```python
from build123d import *

# Parameters (mm, degrees)
SKETCH2_W           = 226.3
SKETCH2_H           = 100
BOSS_EXTRUDE1_DEPTH = 183
SKETCH4_OUTSIDE_W   = 316.656
SKETCH4_OUTSIDE_H   = 190.356
SKETCH4_OUTSIDE_W_2 = 8.5
SKETCH4_OUTSIDE_H_2 = 8.5
CUT_EXTRUDE1_DEPTH  = 6
SKETCH5_W           = 209.3
SKETCH5_H           = 114
CUT_EXTRUDE2_DEPTH  = 238.259188442
SKETCH6_W           = 83
SKETCH6_H           = 114
CUT_EXTRUDE3_DEPTH  = 296.29762952
EXTRUDE_THIN1_START = -2.5
EXTRUDE_THIN1_DEPTH = 3.5
EXTRUDE_THIN2_START = -2.5
EXTRUDE_THIN2_DEPTH = 3.5
CIRPATTERN1_COUNT   = 2


with BuildPart() as part:
    # Sketch2 → Boss-Extrude1 (new, symmetric)
    with BuildSketch(Plane(origin=(0, 0, 0), x_dir=(1, 0, 0), z_dir=(0, 1, 0))):
        Rectangle(SKETCH2_W, SKETCH2_H)
    extrude(amount=BOSS_EXTRUDE1_DEPTH, both=True)

    # Sketch4 outside → Cut-Extrude1 (cut)
    with BuildSketch(Plane.XZ.offset(183)):
        Rectangle(SKETCH4_OUTSIDE_W, SKETCH4_OUTSIDE_H)
        with Locations((-108.9, 45.75)):
            Rectangle(SKETCH4_OUTSIDE_W_2, SKETCH4_OUTSIDE_H_2, mode=Mode.SUBTRACT)
        with Locations((-108.9, -45.75)):
            Rectangle(SKETCH4_OUTSIDE_W_2, SKETCH4_OUTSIDE_H_2, mode=Mode.SUBTRACT)
        with Locations((108.9, -45.75)):
            Rectangle(SKETCH4_OUTSIDE_W_2, SKETCH4_OUTSIDE_H_2, mode=Mode.SUBTRACT)
        with Locations((108.9, 45.75)):
            Rectangle(SKETCH4_OUTSIDE_W_2, SKETCH4_OUTSIDE_H_2, mode=Mode.SUBTRACT)
    cut_extrude1 = extrude(amount=-CUT_EXTRUDE1_DEPTH, mode=Mode.SUBTRACT)

    # Mirror1: Cut-Extrude1 across plane
    add(cut_extrude1.mirror(Plane.ZX), mode=Mode.SUBTRACT)

    # Sketch5 → Cut-Extrude2 (cut, through all)
    with BuildSketch(Plane.XY.offset(50)):
        with Locations((0, 117)):
            Rectangle(SKETCH5_W, SKETCH5_H)
        with Locations((0, -117)):
            Rectangle(SKETCH5_W, SKETCH5_H)
        Rectangle(SKETCH5_W, SKETCH5_H)
    extrude(amount=-CUT_EXTRUDE2_DEPTH, mode=Mode.SUBTRACT)

    # Sketch6 → Cut-Extrude3 (cut, through all)
    with BuildSketch(Plane(origin=(113.15, 0, 0), x_dir=(0, 0, -1), z_dir=(1, 0, 0))):
        with Locations((0, 117)):
            Rectangle(SKETCH6_W, SKETCH6_H)
        with Locations((0, -117)):
            Rectangle(SKETCH6_W, SKETCH6_H)
        Rectangle(SKETCH6_W, SKETCH6_H)
    extrude(amount=-CUT_EXTRUDE3_DEPTH, mode=Mode.SUBTRACT)

    # Sketch7 → Extrude-Thin1 (add)
    with BuildSketch(Plane.XY.offset(50).offset(EXTRUDE_THIN1_START)):
        Polygon((-103.812934943, -175.536822075), (105.487065057, -61.536822075), (103.812934943, -58.463177925), (-105.487065057, -172.463177925), align=None)
        Polygon((-103.812934943, -58.536822075), (105.487065057, 55.463177925), (103.812934943, 58.536822075), (-105.487065057, -55.463177925), align=None)
        Polygon((-103.812934943, 58.463177925), (105.487065057, 172.463177925), (103.812934943, 175.536822075), (-105.487065057, 61.536822075), align=None)
    extrude_thin1 = extrude(amount=-EXTRUDE_THIN1_DEPTH)

    # Sketch8 → Extrude-Thin2 (add)
    with BuildSketch(Plane(origin=(113.15, 0, 0), x_dir=(0, 0, -1), z_dir=(1, 0, 0)).offset(EXTRUDE_THIN2_START)):
        Polygon((-40.085248698, -175.030038229), (42.914751302, -61.030038229), (40.085248698, -58.969961771), (-42.914751302, -172.969961771), align=None)
        Polygon((-40.085248698, -58.030038229), (42.914751302, 55.969961771), (40.085248698, 58.030038229), (-42.914751302, -55.969961771), align=None)
        Polygon((-40.085248698, 58.969961771), (42.914751302, 172.969961771), (40.085248698, 175.030038229), (-42.914751302, 61.030038229), align=None)
    extrude_thin2 = extrude(amount=-EXTRUDE_THIN2_DEPTH)

    # CirPattern1: Extrude-Thin1, Extrude-Thin2 ×2 about axis
    cirpattern1_axis = Axis((0, 0, 0), (0, 1, 0))
    add([extrude_thin1.rotate(cirpattern1_axis, i * 360 / CIRPATTERN1_COUNT) for i in range(1, CIRPATTERN1_COUNT)])
    add([extrude_thin2.rotate(cirpattern1_axis, i * 360 / CIRPATTERN1_COUNT) for i in range(1, CIRPATTERN1_COUNT)])


solid = part.part
```
Geometry: final body of the model. Coordinates: model frame, mm. A direction names the side the tool comes from. Coordinates: 2 decimals unless noted, no trailing zeros. Answer in a Markdown table with one row per item. Add a question column.
Q1. Mould query, pull axis Z, two halves, no side actions, for faces 1 (the flat face through (-108.92, 114.74, 0.52)), 2 (the flat face through (0, 117, -47.5)), 3 (the flat face through (-0.39, 118.78, 45.77)). Classes: released by +Z, released by -Z, zero draft, split by the parting line, or undercut.
Q2. Section query A-A on y = 137.5. Count the separate pieces of the cut face and the enclosed holes in it, and give its area (3 significant figures).
Q3. Contact query for flat-ended pins moving along their axis: P1, Ø3, axis at x = 88.5, z = -15, coming from the +Y side; P2, Ø1, axis at x = -9, z = 32.5, coming from the -Y side; P3, Ø4, axis at y = 3, z = -1, coming from the +X side. Output: stop coordinate, or through.
Q4. Reachability of faces 4 (the flat face through (-109, -183, 46)), 5 (the flat face through (110.65, -117, 0)) from +Z, -Z, +X, -X, +Y, -Y: full face, straight path, thin tool, end or side. Return the list, or none.
Q5. Line query: L1, parallel to Y at x = 61.5, z = -9.5; L2, parallel to X at y = 80.5, z = 27.5; L3, parallel to X at y = 26.5, z = -42. Output: solid intervals per line, ascending.
Completed:
| question | item | result |
|---|---|---|
| 1 | face 1 | undercut |
| 1 | face 2 | released by -Z |
| 1 | face 3 | zero draft |
| 2 | separate pieces | 8 |
| 2 | enclosed holes | 0 |
| 2 | area | 371 mm2 |
| 3 | P1 | stops at y = 177 |
| 3 | P2 | stops at y = -177 |
| 3 | P3 | stops at x = 110.65 |
| 4 | face 4 | +Z, -Z, +X, -X, -Y |
| 4 | face 5 | +X |
| 5 | L1 | y = -177 to -174, -60 to -57, 57 to 60, 174 to 177 |
| 5 | L2 | x = 107.15 to 110.65 |
| 5 | L3 | x = -113.15 to -104.65, 104.65 to 113.15 |
